Input: dimensioned drawing with shaded views. Units: mm. Origin: part minimum x, y, z. Coordinates: 2 decimals unless noted, no trailing zeros. Loops run counter-clockwise (first coordinate to the right, second up) from the corner with the lowest first, then second, coordinate; pieces in that order, holes last. Notation, with made-up numbers: (-21, 56) - (27, 56) arc R10 ccw to (27, 69) - close; hole circle Ø11 at (61.25, -39). An arc over 180 degrees is marked (long way). Use one line per item in the form item = value. Start each with the question number.
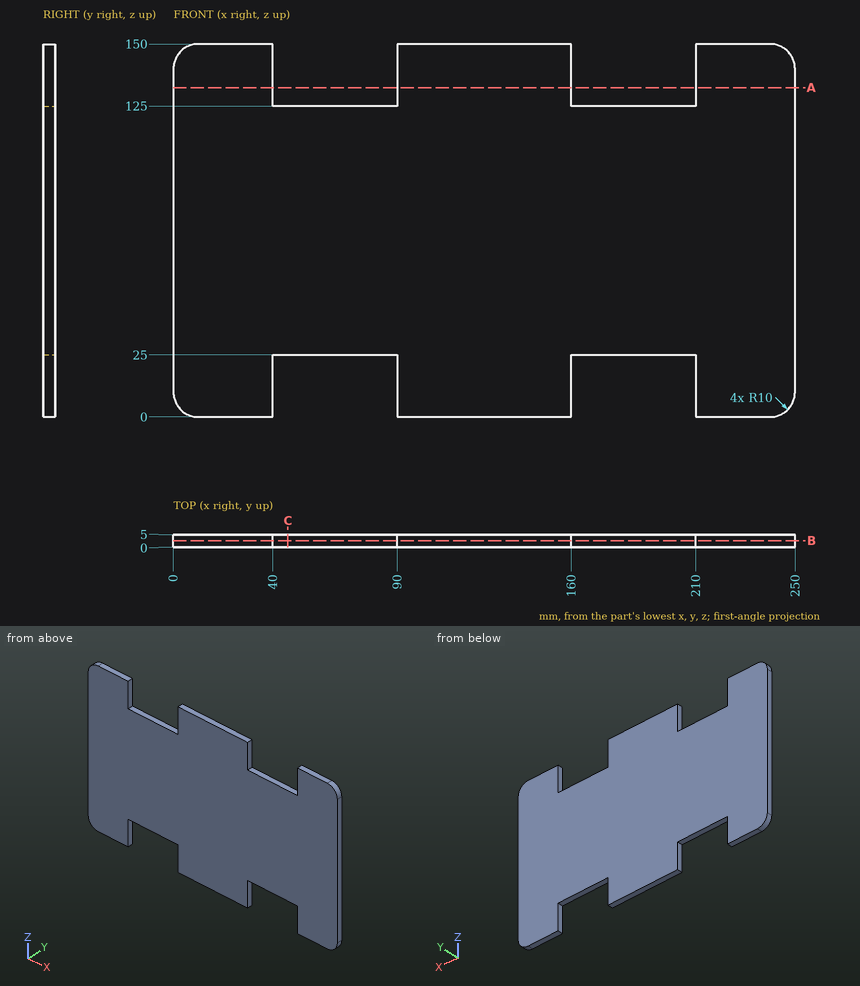
(1) Cut plane B-B, the plane y = 2.75. Output: boundary loops of the cut face in (x, z), plus the area to 3 significant figures.
(2) Cut plane A-A, the plane z = 132.5. Output: boundary loops of the cut face in (x, y).
(3) Cut plane C-C, the plane x = 46. Output: boundary loops of the cut face in (y, z), plus the area to 3 significant figures.
(4) Contact query for flat-ended pins moving along their axis: pin 1 (3 mm diameter, centred on x = 85.5, y = 3.5, fed in from -Z); pin 2 (2.5 mm diameter, centred on x = 77, y = 1.5, fed in from +Z). Output: stop coordinate, or through.
(5) Material intervals for line 1 (X direction, y = 2.55, z = 133); line 2 (Z direction, x = 170.5, y = 2.85), sorted ascending.
Recorded:
q1.outline = (0, 10) arc R10 ccw to (10, 0) - (40, 0) - (40, 25) - (90, 25) - (90, 0) - (160, 0) - (160, 25) - (210, 25) - (210, 0) - (240, 0) arc R10 ccw to (250, 10) - (250, 140) arc R10 ccw to (240, 150) - (210, 150) - (210, 125) - (160, 125) - (160, 150) - (90, 150) - (90, 125) - (40, 125) - (40, 150) - (10, 150) arc R10 ccw to (0, 140) - close
q1.area = 32,400 mm²
q2.outline = (0, 0) - (40, 0) - (40, 5) - (0, 5) - close; (90, 0) - (160, 0) - (160, 5) - (90, 5) - close; (210, 0) - (250, 0) - (250, 5) - (210, 5) - close
q3.outline = (0, 25) - (5, 25) - (5, 125) - (0, 125) - close
q3.area = 500 mm²
q4.pin_1 = 25
q4.pin_2 = 125
q5.line_1 = 0 to 40, 90 to 160, 210 to 250
q5.line_2 = 25 to 125
